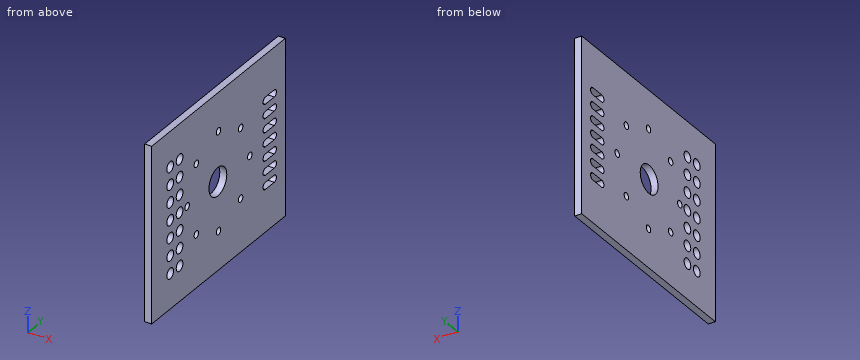
```python
from build123d import *

# Parameters (mm, degrees)
SKETCH_1_W      = 250
SKETCH_1_H      = 300
SKETCH_1_R      = 20
SKETCH_1_R_2    = 7.5
SKETCH_1_R_3    = 5
EXTRUDE_2_DEPTH = 10


with BuildPart() as part:
    # 草图1 → 凸台-拉伸2 (new body)
    with BuildSketch(Plane(origin=(0, 0, 0), x_dir=(0, 0, -1), z_dir=(1, 0, 0))):
        Rectangle(SKETCH_1_W, SKETCH_1_H)
        with Locations((0, -1.426013128)):
            Circle(SKETCH_1_R, mode=Mode.SUBTRACT)
        with Locations((0, -87.366817617)):
            Circle(SKETCH_1_R_2, mode=Mode.SUBTRACT)
        with Locations((0, 70.265)):
            Circle(SKETCH_1_R_3, mode=Mode.SUBTRACT)
        with Locations((49.68485798, 49.68485798)):
            Circle(SKETCH_1_R_3, mode=Mode.SUBTRACT)
        with Locations((70.265, 0)):
            Circle(SKETCH_1_R_3, mode=Mode.SUBTRACT)
        with Locations((49.68485798, -49.68485798)):
            Circle(SKETCH_1_R_3, mode=Mode.SUBTRACT)
        with Locations((0, -70.265)):
            Circle(SKETCH_1_R_3, mode=Mode.SUBTRACT)
        with Locations((-49.68485798, -49.68485798)):
            Circle(SKETCH_1_R_3, mode=Mode.SUBTRACT)
        with Locations((-70.265, 0)):
            Circle(SKETCH_1_R_3, mode=Mode.SUBTRACT)
        with Locations((-49.68485798, 49.68485798)):
            Circle(SKETCH_1_R_3, mode=Mode.SUBTRACT)
        with Locations((0, -108.413247163)):
            Circle(SKETCH_1_R_2, mode=Mode.SUBTRACT)
        with Locations((25, -87.366817617)):
            Circle(SKETCH_1_R_2, mode=Mode.SUBTRACT)
        with Locations((25, -108.413247163)):
            Circle(SKETCH_1_R_2, mode=Mode.SUBTRACT)
        with Locations((50, -87.366817617)):
            Circle(SKETCH_1_R_2, mode=Mode.SUBTRACT)
        with Locations((50, -108.413247163)):
            Circle(SKETCH_1_R_2, mode=Mode.SUBTRACT)
        with Locations((75, -87.366817617)):
            Circle(SKETCH_1_R_2, mode=Mode.SUBTRACT)
        with Locations((75, -108.413247163)):
            Circle(SKETCH_1_R_2, mode=Mode.SUBTRACT)
        with Locations((-25, -87.366817617)):
            Circle(SKETCH_1_R_2, mode=Mode.SUBTRACT)
        with Locations((-25, -108.413247163)):
            Circle(SKETCH_1_R_2, mode=Mode.SUBTRACT)
        with Locations((-50, -87.366817617)):
            Circle(SKETCH_1_R_2, mode=Mode.SUBTRACT)
        with Locations((-50, -108.413247163)):
            Circle(SKETCH_1_R_2, mode=Mode.SUBTRACT)
        with Locations((-75, -87.366817617)):
            Circle(SKETCH_1_R_2, mode=Mode.SUBTRACT)
        with Locations((-75, -108.413247163)):
            Circle(SKETCH_1_R_2, mode=Mode.SUBTRACT)
        with BuildLine():
            Line((5, 125), (5, 105))
            ThreePointArc((5, 105), (0, 100), (-5, 105))
            Line((-5, 105), (-5, 125))
            ThreePointArc((-5, 125), (0, 130), (5, 125))
        make_face(mode=Mode.SUBTRACT)
        with BuildLine():
            Line((25, 125), (25, 105))
            ThreePointArc((25, 105), (20, 100), (15, 105))
            Line((15, 105), (15, 125))
            ThreePointArc((15, 125), (20, 130), (25, 125))
        make_face(mode=Mode.SUBTRACT)
        with BuildLine():
            Line((45, 125), (45, 105))
            ThreePointArc((45, 105), (40, 100), (35, 105))
            Line((35, 105), (35, 125))
            ThreePointArc((35, 125), (40, 130), (45, 125))
        make_face(mode=Mode.SUBTRACT)
        with BuildLine():
            Line((65, 125), (65, 105))
            ThreePointArc((65, 105), (60, 100), (55, 105))
            Line((55, 105), (55, 125))
            ThreePointArc((55, 125), (60, 130), (65, 125))
        make_face(mode=Mode.SUBTRACT)
        with BuildLine():
            Line((-15, 125), (-15, 105))
            ThreePointArc((-15, 105), (-20, 100), (-25, 105))
            Line((-25, 105), (-25, 125))
            ThreePointArc((-25, 125), (-20, 130), (-15, 125))
        make_face(mode=Mode.SUBTRACT)
        with BuildLine():
            Line((-35, 125), (-35, 105))
            ThreePointArc((-35, 105), (-40, 100), (-45, 105))
            Line((-45, 105), (-45, 125))
            ThreePointArc((-45, 125), (-40, 130), (-35, 125))
        make_face(mode=Mode.SUBTRACT)
        with BuildLine():
            Line((-55, 125), (-55, 105))
            ThreePointArc((-55, 105), (-60, 100), (-65, 105))
            Line((-65, 105), (-65, 125))
            ThreePointArc((-65, 125), (-60, 130), (-55, 125))
        make_face(mode=Mode.SUBTRACT)
    extrude(amount=EXTRUDE_2_DEPTH)


solid = part.part
```
Can you work these out from the model? Positions are in its coordinate system, mm. Give positions to 0.01 mm unless a question says otherwise; leave off trailing zeros. Write each loop counter-clockwise with the first axis right and the second up, starting at its lowest first coordinate (ties: lowest second). Pieces come first, ordered by that corner, then holes. Notation, with made-up numbers: (37, 61.25) - (60, 61.25) arc R9 cw to (60, 68.25) - close; hole circle Ø6 at (-10.75, 70). An arc over 180 degrees is marked (long way). Write item = value, one per line. Start each with the question number.
1. Imagine slicing it at A-A (y = 118). Count the separate pieces of the cut face and the enclosed holes in it, and give its area (3 significant figures).
2. Please list where these lines run through material, in increasing order: line 1 (Y direction, x = 1, z = -80); line 2 (Y direction, x = 8.25, z = -23); line 3 (Y direction, x = 9, z = -69.5).
3. Imagine slicing it at B-B (z = -50). Please give me the cut outline in (x, y).
Worked answers:
q1.separate_pieces = 8
q1.enclosed_holes = 0
q1.area = 1,800 mm2
q2.line_1 = -150 to -114, -102.82 to -92.96, -81.78 to 150
q2.line_2 = -150 to -115.64, -101.18 to -94.6, -80.14 to 101, 129 to 150
q2.line_3 = -150 to -113.51, -103.31 to -92.47, -82.27 to -4.94, 4.94 to 150
q3.outline = (0, -150) - (10, -150) - (10, -115.91) - (0, -115.91) - close; (0, -100.91) - (10, -100.91) - (10, -94.87) - (0, -94.87) - close; (0, -79.87) - (10, -79.87) - (10, -54.67) - (0, -54.67) - close; (0, -44.69) - (10, -44.69) - (10, 44.69) - (0, 44.69) - close; (0, 54.67) - (10, 54.67) - (10, 150) - (0, 150) - close
